```python
from build123d import *

# Parameters (mm, degrees)
BOSS_EXTRUDE1_DEPTH = 2
SCALE1_SCALE        = 1.4
SKETCH2_R           = 1.5
CUT_EXTRUDE1_DEPTH  = 3.8
SKETCH3_R           = 1.5
CUT_EXTRUDE2_DEPTH  = 3.8


with BuildPart() as part:
    # Sketch1 → Boss-Extrude1 (new body)
    with BuildSketch(Plane(origin=(0, 0, 0), x_dir=(1, 0, 0), z_dir=(0, 1, 0))):
        Polygon((1.719047443, 61.234571581), (-10.280952557, 61.234571581), (-15.280952557, 52.574317544), (-15.280952557, 10.574317544), (-7.901694864, -38.292126086), (4.105557327, -38.292126086), (4.105557327, 1.707873914), (6.719047443, 6.234571581), (6.719047443, 56.234571581), align=None)
    extrude(amount=BOSS_EXTRUDE1_DEPTH)


with BuildPart() as part_1:
    # Scale1: scaled about (-3.98494468, 1, -15.536034959)
    add(part.part.scale(SCALE1_SCALE).moved(Location((1.593977872, -0.4, 6.214413984))))

    # Sketch2 → Cut-Extrude1 (cut, through all)
    with BuildSketch(Plane(origin=(0, 2.4, 0), x_dir=(1, 0, 0), z_dir=(0, 1, 0))):
        with Locations((-3.999355707, 14.51398623)):
            Circle(SKETCH2_R)
        with Locations((-3.999355707, 58.51398623)):
            Circle(SKETCH2_R)
    extrude(amount=-CUT_EXTRUDE1_DEPTH, mode=Mode.SUBTRACT)

    # Sketch3 → Cut-Extrude2 (cut, through all)
    with BuildSketch(Plane(origin=(0, 2.4, 0), x_dir=(1, 0, 0), z_dir=(0, 1, 0))):
        with Locations((-1.658241871, -46.323390503)):
            Circle(SKETCH3_R)
        with Locations((-1.658241871, -54.323390503)):
            Circle(SKETCH3_R)
    extrude(amount=-CUT_EXTRUDE2_DEPTH, mode=Mode.SUBTRACT)


solid = part_1.part
```
Could you check a few things on this model? Use its own coordinates, in mm. Round coordinates to 2 decimals unless told otherwise and drop trailing zeros. Write each loop counter-clockwise with the first axis right and the second up, starting at its lowest first coordinate (ties: lowest second). Pieces come first, ordered by that corner, then holes. Notation, with made-up numbers: M 50,-28.75 L 98,-28.75 A19 cw 98,-1.75 Z; hole C -13.5,2.5 d9. An arc over 180 degrees is marked long. Answer in a Markdown table with one row per item. Add a question column.
Q1. If I drill on line 1 (Z direction, x = -3.5, y = 0.1); line 2 (Z direction, x = -3, y = 2.15); line 3 (Z direction, x = 8.5, y = 0.9), over which ranges is the centre line in solid material (lowest first)? Write a range as from..to.
Q2. If we mould it in two halves opening along Z, with no side actions, what happens to faces 1 (the cylindrical face through (-1.854, 1.02, 52.836)), 2 (the flat face through (-14.706, 0.98, 25.138)), 3 (the cylindrical face through (-5.498, 1.02, -14.58)), 4 (the flat face through (7.342, 1, 32))? For each: +Z half, -Z half, draft (parallel to the pull), parting line (faces both ways), or undercut.
Q3. Imagine slicing it at C-C (x = 9.5). Please give me the cut outline in (y, z).
Q4. Imagine slicing it at B-B (z = 24). Please give me the cut outline in (x, y).
Q5. Imagine slicing it at A-A (y = 0.85). Please give me the cut outline in (x, z), then the cut area to 3 significant figures.
Values:
| question | item | result |
|---|---|---|
| 1 | line 1 | -79.51..-59.93, -57.1..-15.93, -13.1..59.82 |
| 1 | line 2 | -79.51..-59.63, -57.4..-15.63, -13.4..45.65, 46.99..53.65, 54.99..59.82 |
| 1 | line 3 | -75.01..1.82 |
| 2 | face 1 | undercut |
| 2 | face 2 | +Z half |
| 2 | face 3 | undercut |
| 2 | face 4 | draft |
| 3 | outline | M -0.4,-74.01 L 2.4,-74.01 L 2.4,0.09 L -0.4,0.09 Z |
| 4 | outline | M -14.88,-0.4 L 7.34,-0.4 L 7.34,2.4 L -14.88,2.4 Z |
| 5 | outline | M -19.8,-67.39 L -12.8,-79.51 L 4,-79.51 L 11,-72.51 L 11,-2.51 L 7.34,3.82 L 7.34,59.82 L -9.47,59.82 L -19.8,-8.59 Z; hole C -4,-58.51 d3; hole C -4,-14.51 d3; hole C -1.66,46.32 d3; hole C -1.66,54.32 d3 |
| 5 | area | 3,630 mm^2 |
